Could you check a few things on this model? Use its own coordinates, in mm. Face numbers are marked on the shaded views. A direction names the side the tool comes from. Give positions to 0.01 mm unless a question says otherwise; leave off trailing zeros. Loops run counter-clockwise (first coordinate to the right, second up) from the corner with the lowest first, then second, coordinate; pieces in that order, holes last. Notation, with made-up numbers: (40.5, 8) - (74.5, 8) arc R20 cw to (74.5, 44) - close; hole circle Ø6 at (12, 41.5). An arc over 180 degrees is marked (long way). One line per item, written item: value. Start each with the question number.
Q1. I want a section at B-B (x = -15.5). Please give me the cut outline in (y, z).
Q2. I want a section at A-A (y = 16). Please give me the cut outline in (x, z), then the cut area to 3 significant figures.
Q3. For the marked faces 1, 2, 3, 4 and 5, which set-ups out of +Z, -Z, +X, -X, +Y, -Y let a thin tool reach every point of the face, with its end or its side?
Q4. I'm going to push flat-ended pins straight in: P1, Ø12, axis at x = -45, y = 30, coming from the +Z side; P2, Ø6, axis at x = -47.5, y = 28, coming from the -Z side; P3, Ø3, axis at y = 27, z = 4, coming from the -X side; P4, Ø8, axis at x = -43, z = 37.5, coming from the +Y side. Where does each tip first touch, or does it pass through?
Q5. If I drill on line 1 (Y direction, x = -14.5, z = 9.5); line 2 (Z direction, x = -36.5, y = 13); line 3 (X direction, y = 12, z = 31), over which ranges is the centre line in solid material (lowest first)? Write a range as from..to.
Q6. I want a section at D-D (x = -35). Please give me the cut outline in (y, z).
Q7. If we mould it in two halves opening along Z, with no side actions, what happens to the marked faces 6, 7 and 8? For each: released by +Z, released by -Z, zero draft, split by the parting line, or undercut.
Q8. I want a section at C-C (z = 3). Please give me the cut outline in (x, y).
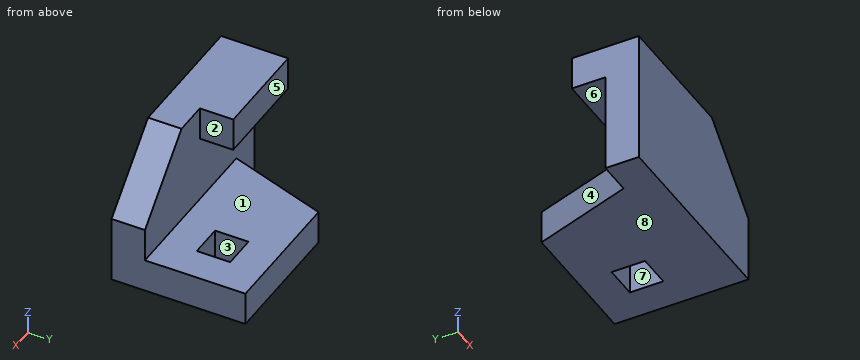
Autodesk Inventor part; units mm, degrees
ref_plane "YZ Plane" through (0, 0, 0) normal (1, 0, 0) x (0, 1, 0)
ref_plane "XZ Plane" through (0, 0, 0) normal (0, 1, 0) x (-1, 0, 0)
ref_plane "XY Plane" through (0, 0, 0) normal (0, 0, 1) x (1, 0, 0)
sketch "草圖1" plane through (0, 0, 0) normal (0, 1, 0) x (-1, 0, 0)
  line L0 (0, 0) -> (60, 0)
  line L1 (60, 0) -> (60, 40)
  line L2 (60, 40) -> (0, 40)
  line L3 (0, 40) -> (0, 0)
  line L4 (20, 40) -> (0, 20)
  dimension "d0" = 60
  dimension "d1" = 40
  dimension "d2" = 20
  dimension "d3" = 20
extrude "擠出1" add sketch "草圖1" along normal blind 10 contours L3 L4 L2 L1 L0
sketch "草圖2" plane through (0, 0, 0) normal (0, 0, -1) x (-1, 0, 0)
  line L0 (0, 0) -> (0, 10)
  line L1 (0, 10) -> (60, 10)
  line L2 (60, 10) -> (60, 0)
  line L3 (60, 0) -> (0, 0)
  line L4 (50, 10) -> (40, 40)
  line L5 (40, 40) -> (0, 40)
  line L6 (0, 40) -> (0, 10)
  line L7 (20, 30) -> (10, 30)
  line L8 (10, 30) -> (10, 20)
  line L9 (10, 20) -> (20, 20)
  line L10 (20, 20) -> (20, 30)
  dimension "d6" = 10
  dimension "d7" = 40
  dimension "d8" = 40
  dimension "d9" = 10
  dimension "d10" = 10
  dimension "d11" = 10
extrude "擠出2" add sketch "草圖2" against normal blind 10 contours L6 L5 L4 L1
sketch "草圖3" plane through (0, 10, 0) normal (0, 1, 0) x (1, 0, 0)
  line L0 (-20, -40) -> (-60, -40)
  line L1 (-60, -40) -> (-60, 0)
  line L2 (-60, 0) -> (-50, 0)
  line L3 (-50, -10) -> (-50, 0)
  line L4 (0, -10) -> (-50, -10)
  line L5 (0, 0) -> (0, -10)
  line L6 (-50, 0) -> (0, 0)
  line L7 (0, -20) -> (-20, -40)
  line L8 (0, -10) -> (0, -20)
  line L9 (-60, 0) -> (-60, -40)
  line L10 (-60, -40) -> (-30, -40)
  line L11 (-30, -40) -> (-30, -30)
  line L12 (-30, -30) -> (-60, -30)
  line L13 (-60, -30) -> (-60, -40)
  dimension "d14" = 10
  dimension "d15" = 30
extrude "擠出3" add sketch "草圖3" along normal blind 10 contours L0 L1 L12 L11
properties part number "12" material "鋼、碳鋼"
Worked answers:
1. outline: (0, 0) - (20, 0) - (20, 10) - (10, 10) - (10, 35.5) - (0, 35.5) - close; (30, 0) - (40, 0) - (40, 10) - (30, 10) - close
2. outline: (-60, 30) - (-30, 30) - (-30, 40) - (-60, 40) - close; (-48, 0) - (0, 0) - (0, 10) - (-48, 10) - close
2. area: 780 mm²
3. face 1: +X, -X, +Y
3. face 2: +Z, +X, +Y
3. face 3: +Z, -Z
3. face 4: -Z, -X, +Y
3. face 5: +Z, +X, -X, +Y
4. P1: stops at z = 10
4. P2: passes through
4. P3: stops at x = -44.83
4. P4: stops at y = 20
5. line 1: y = 0..20, 30..40
5. line 2: z = 0..10, 30..40
5. line 3: x = -60..-30
6. outline: (0, 0) - (40, 0) - (40, 10) - (10, 10) - (10, 30) - (20, 30) - (20, 40) - (0, 40) - close
7. face 6: undercut
7. face 7: zero draft
7. face 8: released by -Z
8. outline: (-60, 0) - (0, 0) - (0, 40) - (-40, 40) - (-50, 10) - (-60, 10) - close; hole (-20, 20) - (-10, 20) - (-10, 30) - (-20, 30) - close
